Answer from the drawing. Dimensions are ordinates in mm from the lowest x, y and z of the part. A direction names the side the tool comes from. Round coordinates to 2 decimals unless told otherwise and drop trailing zeros. Write each loop counter-clockwise with the first axis right and the second up, starting at its lowest first coordinate (ties: lowest second). Pieces come first, ordered by that corner, then holes. Notation, with made-up numbers: M 70.5,38.5 L 118.5,38.5 A35 ccw 118.5,72.5 Z; hole C 83,30.5 d1. An arc over 180 degrees is marked long. One line per item, written item: value. Start each with the question number.
(1) For a pull along X with two mould halves and no side action, classify the marked faces 1, 2, 3 and 4 as released by +X, released by -X, zero draft, split by the parting line, or undercut.
(2) Section B-B (z = 2) is taken. Determine the outline of the cut face in (x, y).
(3) For the marked faces 5, 6 and 7, determine the directions among +Z, -Z, +X, -X, +Y, -Y from which every point of the face is accessible in a straight line to the end or side of a thin tool.
(4) Section C-C (y = 7) is taken. Determine the outline of the cut face in (x, z), plus the area to 3 significant figures.
(5) Consider probe 1 along X at (y, z) = (5.5, 7); probe 2 along X at (y, z) = (5.25, 2.5); probe 3 along Y at (x, z) = (6.5, 13.5). Determine where each line is inside the solid, lowest interval first.
(6) Section D-D (x = 5.5) is taken. Determine the outline of the cut face in (y, z).
(7) Section A-A (y = 4.5) is taken. Determine the outline of the cut face in (x, z).
(8) Given P1, Ø3, axis at x = 10, z = 4.5, coming from the -Y side; P2, Ø2, axis at y = 8, z = 1, coming from the +X side; P3, Ø1.1, axis at x = 9, z = 1, coming from the -Y side, each flat-ended and moving along its own axis, determine where each tip first touches the part or whether it passes through.
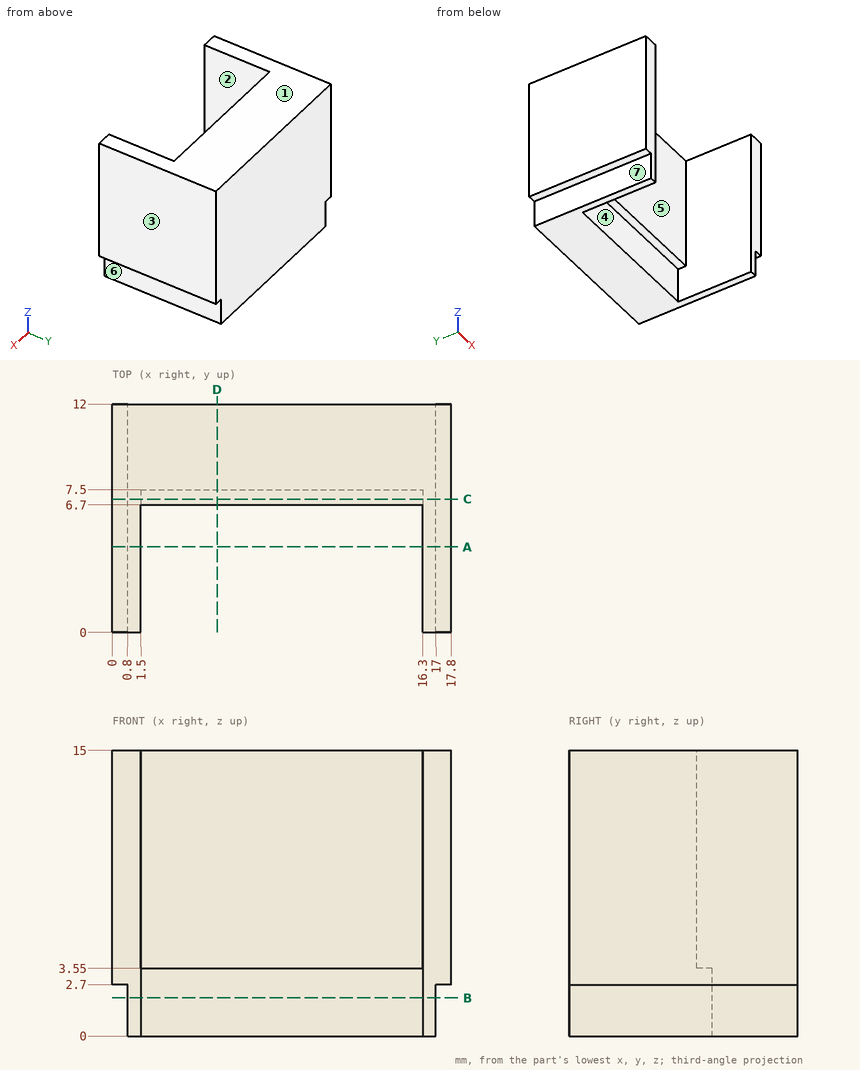
Recorded:
1. face 1: zero draft
1. face 2: undercut
1. face 3: released by +X
1. face 4: undercut
2. outline: M 0.8,0 L 1.5,0 L 1.5,7.5 L 16.3,7.5 L 16.3,0 L 17,0 L 17,12 L 0.8,12 Z
3. face 5: +Z, -Z, -Y
3. face 6: -Z, +X, +Y, -Y
3. face 7: -Z, -X, +Y, -Y
4. outline: M 0,2.7 L 0.8,2.7 L 0.8,0 L 1.5,0 L 1.5,3.55 L 16.3,3.55 L 16.3,0 L 17,0 L 17,2.7 L 17.8,2.7 L 17.8,15 L 0,15 Z
4. area: 210 mm2
5. probe 1: x = 0 to 1.5, 16.3 to 17.8
5. probe 2: x = 0.8 to 1.5, 16.3 to 17
5. probe 3: y = 6.7 to 12
6. outline: M 6.7,3.55 L 7.5,3.55 L 7.5,0 L 12,0 L 12,15 L 6.7,15 Z
7. outline: M 0,2.7 L 0.8,2.7 L 0.8,0 L 1.5,0 L 1.5,15 L 0,15 Z; M 16.3,0 L 17,0 L 17,2.7 L 17.8,2.7 L 17.8,15 L 16.3,15 Z
8. P1: stops at y = 6.7
8. P2: stops at x = 17
8. P3: stops at y = 7.5
